Design review of the part built by this model. Coordinates are the model's own, in mm. Coordinates: 2 decimals unless noted, no trailing zeros. Loops run counter-clockwise (first coordinate to the right, second up) from the corner with the lowest first, then second, coordinate; pieces in that order, holes last. Notation, with made-up numbers: (17, 69) -> (43, 69) arc R19 ccw to (43, 81) -> close; hole circle Ø1 at (24.25, 70). An arc over 180 degrees is marked (long way). Use one line per item in the form item = value. Start each with the question number.
1. The part is to be moulded in two halves that separate along X. For faces 1 (the face through (-12.697, -0.279, 3.131)), 2 (the face through (121.917, 0.279, 3.131)), 3 (the face through (54, 0, 0)), 4 (the face through (-0.69, 3.1, 3.13)), say which applies: released by +X, released by -X, zero draft, split by the parting line, or undercut.
2. Consider section C-C (y = -9.75). State the section outline as (x, z) points.
3. For pin 1 (1 mm diameter, centred on y = 4, z = 2.5, fed in from -X); pin 2 (5 mm diameter, centred on x = 109.22, y = 0, fed in from +Z); pin 3 (3 mm diameter, centred on y = -2.5, z = 3.5, fed in from -X), all flat-tipped, find the tip position at first contact; note any pin that passes through.
4. Consider section B-B (y = 0). State the section outline as (x, z) points (3 decimals), then the cut area to 3 significant figures.
5. Consider section D-D (y = 8.25). State the section outline as (x, z) points.
6. Wall thickness on line 1 (X direction, y = 1.25, z = 6); line 2 (Y direction, x = 109.22, z = 3.25) (3 decimals); line 3 (X direction, y = 0.5, z = 5.25): over which ranges is each line inside the solid? List them lowest first. Write a range as from..to.
7. Consider section A-A (z = 1.5). State the section outline as (x, y) points (3 decimals), then the cut area to 3 significant figures.
Autodesk Inventor part; units mm, degrees
ref_plane "YZ Plane" through (0, 0, 0) normal (1, 0, 0) x (0, 1, 0)
ref_plane "XZ Plane" through (0, 0, 0) normal (0, 1, 0) x (-1, 0, 0)
ref_plane "XY Plane" through (0, 0, 0) normal (0, 0, 1) x (1, 0, 0)
sketch "Sketch1" plane through (0, 0, 0) normal (0, 0, 1) x (1, 0, 0)
  line L0 (0, 0) -> (109.22, 0) construction
  line L1 (0, -12.7) -> (109.22, -12.7)
  line L2 (109.22, 12.7) -> (0, 12.7)
  arc A0 (0, 12.7) -> (0, -12.7) centre (0, 0) ccw
  arc A1 (109.22, -12.7) -> (109.22, 12.7) centre (109.22, 0) ccw
  circle A2 centre (0, 0) radius 3.175
  circle A3 centre (109.22, 0) radius 3.175
  point P0 (54.61, 0)
  dimension "d0" = 25.4
  dimension "d1" = 109.22
  dimension "d2" = 6.35
extrude "Extrusion1" add sketch "Sketch1" along normal blind 6.35
properties part number "ScissorHookBar"
Geometry check:
q1.face_1 = released by -X
q1.face_2 = released by +X
q1.face_3 = zero draft
q1.face_4 = undercut
q2.outline = (-8.14, 0) -> (117.36, 0) -> (117.36, 6.35) -> (-8.14, 6.35) -> close
q3.pin_1 = -12.21
q3.pin_2 = through
q3.pin_3 = -12.66
q4.outline = (-12.7, 0) -> (-3.175, 0) -> (-3.175, 6.35) -> (-12.7, 6.35) -> close; (3.175, 0) -> (106.045, 0) -> (106.045, 6.35) -> (3.175, 6.35) -> close; (112.395, 0) -> (121.92, 0) -> (121.92, 6.35) -> (112.395, 6.35) -> close
q4.area = 774 mm²
q5.outline = (-9.66, 0) -> (118.88, 0) -> (118.88, 6.35) -> (-9.66, 6.35) -> close
q6.line_1 = -12.64..-2.92, 2.92..106.3, 112.14..121.86
q6.line_2 = -12.7..-3.175, 3.175..12.7
q6.line_3 = -12.69..-3.14, 3.14..106.08, 112.36..121.91
q7.outline = (0, -12.7) -> (109.22, -12.7) arc R12.7 ccw to (109.22, 12.7) -> (0, 12.7) arc R12.7 ccw to start; hole circle Ø6.35 at (0, 0); hole circle Ø6.35 at (109.22, 0)
q7.area = 3,220 mm²
